Autodesk Inventor part; units mm, degrees
ref_plane "YZ Plane" through (0, 0, 0) normal (1, 0, 0) x (0, 1, 0)
ref_plane "XZ Plane" through (0, 0, 0) normal (0, 1, 0) x (-1, 0, 0)
ref_plane "XY Plane" through (0, 0, 0) normal (0, 0, 1) x (1, 0, 0)
sketch "Sketch1" plane through (0, 0, 0) normal (0, 0, 1) x (1, 0, 0)
  circle A0 centre (80.14, 40.64) radius 3.57
  circle A1 centre (40.14, 40.64) radius 2.5
  circle A2 centre (40.14, 50.64) radius 2.5
  circle A3 centre (40.14, 60.64) radius 2.5
  circle A4 centre (40.14, 30.64) radius 2.5
  circle A5 centre (40.14, 20.64) radius 2.5
  circle A6 centre (7.59, 40.64) radius 12.5
  arc A7 (-4.314, 26.544) -> (-6.506, 28.736) centre (-5.41, 27.64) ccw
  line L0 (-6.814, 24.044) -> (-4.314, 26.544)
  arc A8 (-9.006, 26.236) -> (-6.814, 24.044) centre (-7.91, 25.14) ccw
  line L1 (-6.506, 28.736) -> (-9.006, 26.236)
  line L2 (-4.314, 54.736) -> (-6.814, 57.236)
  arc A9 (-6.506, 52.544) -> (-4.314, 54.736) centre (-5.41, 53.64) ccw
  line L3 (-9.006, 55.044) -> (-6.506, 52.544)
  arc A10 (-6.814, 57.236) -> (-9.006, 55.044) centre (-7.91, 56.14) ccw
  line L4 (21.994, 57.236) -> (19.494, 54.736)
  arc A11 (19.494, 54.736) -> (21.686, 52.544) centre (20.59, 53.64) ccw
  line L5 (21.686, 52.544) -> (24.186, 55.044)
  arc A12 (24.186, 55.044) -> (21.994, 57.236) centre (23.09, 56.14) ccw
  line L6 (24.186, 26.236) -> (21.686, 28.736)
  arc A13 (21.686, 28.736) -> (19.494, 26.544) centre (20.59, 27.64) ccw
  line L7 (19.494, 26.544) -> (21.994, 24.044)
  arc A14 (21.994, 24.044) -> (24.186, 26.236) centre (23.09, 25.14) ccw
  circle A15 centre (60.14, 40.64) radius 2.55
  circle A16 centre (60.14, 30.64) radius 2.55
  circle A17 centre (70.14, 40.64) radius 2.5
  circle A18 centre (60.14, 50.64) radius 2.55
  circle A19 centre (50.14, 40.64) radius 2.5
  line L8 (-12.41, 60.64) -> (-12.41, 20.64)
  line L9 (-12.41, 20.64) -> (46.5039, 15.4857)
  line L10 (46.5039, 15.4857) -> (88.14, 30.64)
  line L11 (88.14, 30.64) -> (88.14, 50.64)
  line L12 (88.14, 50.64) -> (46.5039, 65.7943)
  line L13 (46.5039, 65.7943) -> (-12.41, 60.64)
  point P0 (0, 0)
  dimension "d0" = 40
  dimension "d1" = 20
  dimension "d2" = 20
  dimension "d3" = 8
  dimension "d4" = 10
  dimension "d5" = 20
  dimension "d6" = 95
  dimension "d7" = 95
  dimension "d8" = 110
  dimension "d9" = 110
extrude "Extrusion1" add sketch "Sketch1" along normal blind 3
fillet "Fillet1" radius 5 6 edges at (-12.41, 20.64, 1.5) (46.5039, 15.4857, 1.5) (-12.41, 60.64, 1.5) (46.5039, 65.7943, 1.5) (88.14, 50.64, 1.5) (88.14, 30.64, 1.5)
sketch "Sketch2" plane through (0, 0, 0) normal (0, 0, -1) x (-1, 0, 0)
  circle A0 centre (-40.14, 20.64) radius 2.5
  circle A1 centre (-80.14, 40.64) radius 3.57
  circle A2 centre (-40.14, 60.64) radius 2.5
  point P0 (0, 0)
hole "Hole1" at (40.14, 20.64, 0) at (40.14, 60.64, 0) direction (0, 0, 1) diameter 8.1 depth 1
sketch "Sketch3" plane through (0, 0, 0) normal (0, 0, -1) x (-1, 0, 0)
  circle A0 centre (-80.14, 40.64) radius 3.57
  point P0 (0, 0)
hole "Hole2" at (80.14, 40.64, 0) direction (0, 0, 1) diameter 14 depth 1
sketch "Sketch4" plane through (0, 0, 0) normal (0, 0, -1) x (-1, 0, 0)
  circle A0 centre (-80.14, 40.64) radius 7
  circle A1 centre (-40.14, 20.64) radius 4.05
  circle A2 centre (-40.14, 60.64) radius 4.05
  circle A3 centre (-7.59, 40.64) radius 12.5
  circle A4 centre (-60.14, 50.64) radius 2.55
  circle A5 centre (-60.14, 30.64) radius 2.55
  circle A6 centre (-60.14, 40.64) radius 2.55
  circle A7 centre (-50.14, 40.64) radius 2.5
  circle A8 centre (-70.14, 40.64) radius 2.5
  circle A9 centre (-40.14, 30.64) radius 2.5
  circle A10 centre (-40.14, 50.64) radius 2.5
  circle A11 centre (-40.14, 40.64) radius 2.5
  arc A12 (-24.186, 26.236) -> (-21.994, 24.044) centre (-23.09, 25.14) ccw
  line L0 (-24.186, 26.236) -> (-21.686, 28.736)
  arc A13 (-19.494, 26.544) -> (-21.686, 28.736) centre (-20.59, 27.64) ccw
  line L1 (-19.494, 26.544) -> (-21.994, 24.044)
  arc A14 (-21.994, 57.236) -> (-24.186, 55.044) centre (-23.09, 56.14) ccw
  line L2 (-21.994, 57.236) -> (-19.494, 54.736)
  arc A15 (-21.686, 52.544) -> (-19.494, 54.736) centre (-20.59, 53.64) ccw
  line L3 (-21.686, 52.544) -> (-24.186, 55.044)
  arc A16 (4.314, 54.736) -> (6.506, 52.544) centre (5.41, 53.64) ccw
  line L4 (4.314, 54.736) -> (6.814, 57.236)
  arc A17 (9.006, 55.044) -> (6.814, 57.236) centre (7.91, 56.14) ccw
  line L5 (9.006, 55.044) -> (6.506, 52.544)
  line L6 (6.814, 24.044) -> (4.314, 26.544)
  arc A18 (6.506, 28.736) -> (4.314, 26.544) centre (5.41, 27.64) ccw
  line L7 (6.506, 28.736) -> (9.006, 26.236)
  arc A19 (6.814, 24.044) -> (9.006, 26.236) centre (7.91, 25.14) ccw
  arc A20 (-88.14, 34.141) -> (-84.8501, 29.4426) centre (-83.14, 34.141) ccw
  line L8 (-47.5455, 15.8648) -> (-84.8501, 29.4426)
  arc A21 (-47.5455, 15.8648) -> (-45.3997, 15.5823) centre (-45.8354, 20.5633) ccw
  line L9 (7.8458, 20.2407) -> (-45.3997, 15.5823)
  arc A22 (7.8458, 20.2407) -> (12.41, 25.2217) centre (7.41, 25.2217) ccw
  line L10 (12.41, 56.0583) -> (12.41, 25.2217)
  arc A23 (12.41, 56.0583) -> (7.8458, 61.0393) centre (7.41, 56.0583) ccw
  line L11 (-45.3997, 65.6977) -> (7.8458, 61.0393)
  arc A24 (-45.3997, 65.6977) -> (-47.5455, 65.4152) centre (-45.8354, 60.7167) ccw
  line L12 (-84.8501, 51.8374) -> (-47.5455, 65.4152)
  arc A25 (-84.8501, 51.8374) -> (-88.14, 47.139) centre (-83.14, 47.139) ccw
  line L13 (-88.14, 34.141) -> (-88.14, 47.139)
  line L14 (-45.3997, 65.6977) -> (7.8458, 61.0393)
  line L15 (-30.14, 64.3626) -> (-30.14, 16.9174)
  point P0 (0, 0)
  dimension "d27" = 10
extrude "Extrusion2" cut sketch "Sketch4" against normal through all contours L15 L11 A23 L10 A22 L9
fillet "Fillet2" radius 5 2 edges at (30.14, 16.9174, 1.5) (30.14, 64.3626, 1.5)
equation "\"d7\" = d6"
properties part number "2020 Slider" material "Aluminum 6061"
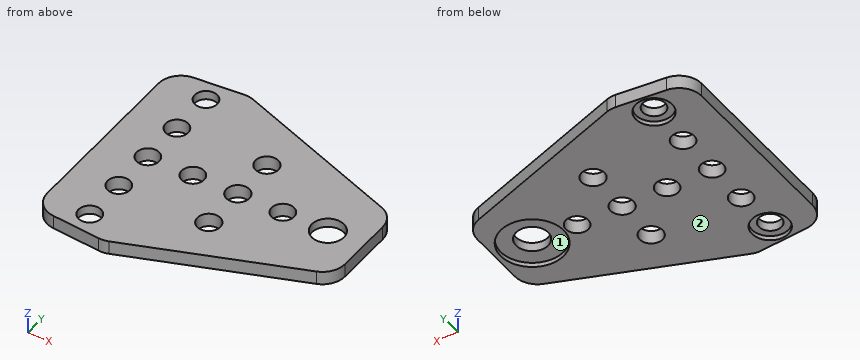
Geometry: final body of the model. Coordinates: model frame, mm. Face numbers are marked on the shaded views. Give positions to 0.01 mm unless a question says otherwise; leave off trailing zeros. Write each loop counter-clockwise with the first axis right and the second up, starting at its lowest first coordinate (ties: lowest second). Pieces come first, ordered by that corner, then holes.
1. Section query C-C, the plane x = 60.14. Return loops of the section in (y, z).
2. Section query D-D, the plane y = 30.64. Return loops of the section in (x, z).
3. Section query B-B, the plane z = 2.45. Count the separate pieces of the cut face and the enclosed holes in it, then the cut area to 3 significant figures.
4. Section query A-A, the plane x = 51. Return loops of the section in (y, z), then the cut area to 3 significant figures.
5. Pin query (flat end, axial travel): P1, Ø2.5, axis at x = 39, y = 19, coming from the -Z side; P2, Ø4.5, axis at x = 70.14, y = 40.64, coming from the -Z side. Return the tip coordinate at first contact, or that it passes through.
6. Draft query along X for the marked faces 1 and 2. Return one class per face: released by +X, released by -X, zero draft, split by the parting line, or undercut.
7. Line query: probe 1 along Y at (x, z) = (40.14, 0.95); probe 2 along Y at (x, z) = (41.5, 1.4); probe 3 along X at (y, z) = (31.5, 1.55). Output: solid intervals per line, ascending.
Computed:
1. outline: (20.45, 0) - (28.09, 0) - (28.09, 3) - (20.45, 3) - close; (33.19, 0) - (38.09, 0) - (38.09, 3) - (33.19, 3) - close; (43.19, 0) - (48.09, 0) - (48.09, 3) - (43.19, 3) - close; (53.19, 0) - (60.83, 0) - (60.83, 3) - (53.19, 3) - close
2. outline: (30.14, 0) - (37.64, 0) - (37.64, 3) - (30.14, 3) - close; (42.64, 0) - (57.59, 0) - (57.59, 3) - (42.64, 3) - close; (62.69, 0) - (86.71, 0) - (86.71, 3) - (62.69, 3) - close
3. separate pieces: 1
3. enclosed holes: 11
3. area: 2,010 mm2
4. outline: (17.12, 0) - (38.29, 0) - (38.29, 3) - (17.12, 3) - close; (42.99, 0) - (64.16, 0) - (64.16, 3) - (42.99, 3) - close
4. area: 127 mm2
5. P1: stops at z = 1
5. P2: passes through
6. face 1: undercut
6. face 2: zero draft
7. probe 1: y = 16.04 to 16.59, 24.69 to 28.14, 33.14 to 38.14, 43.14 to 48.14, 53.14 to 56.59, 64.69 to 65.24
7. probe 2: y = 15.92 to 18.54, 22.74 to 28.54, 32.74 to 38.54, 42.74 to 48.54, 52.74 to 58.54, 62.74 to 65.36
7. probe 3: x = 30.14 to 37.79, 42.49 to 57.74, 62.54 to 87.39
